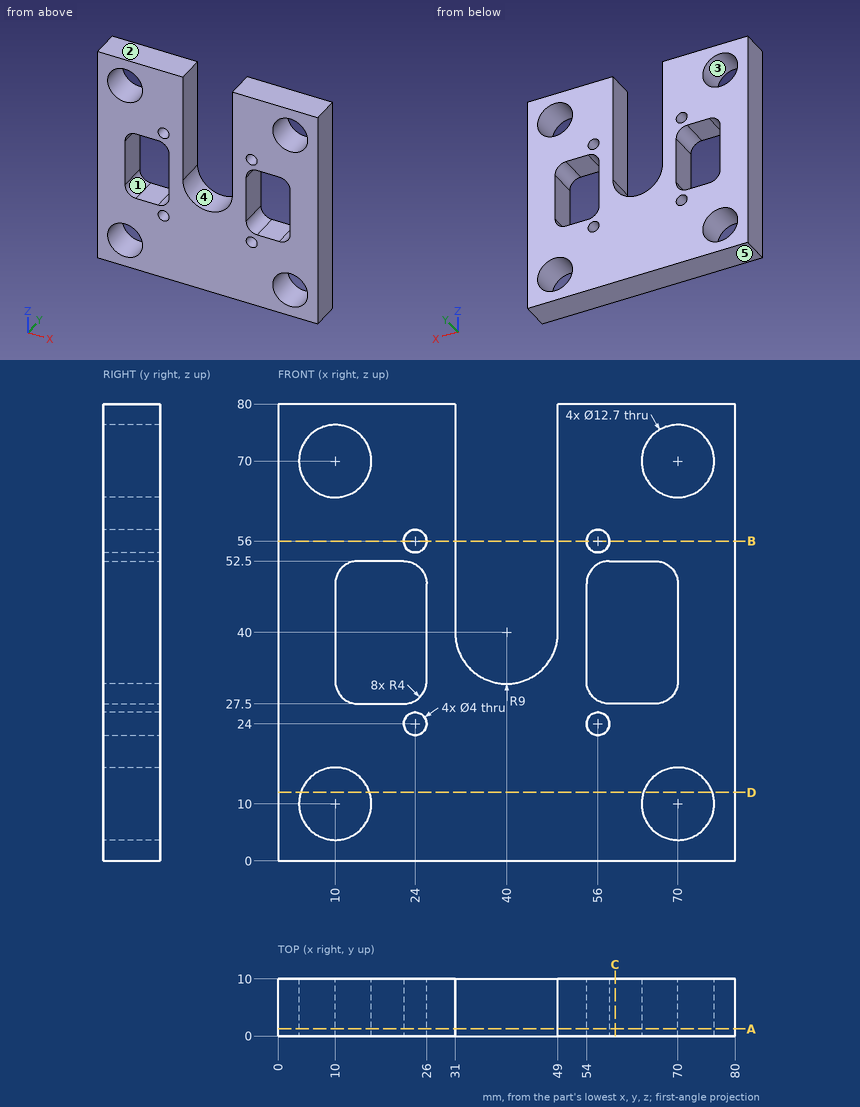
Design review of the part shown in the three views and the two pictorial views. Dimensions are in mm from the part's minimum x, y and z. A direction names the side the tool comes from. Round coordinates to 2 decimals unless told otherwise and drop trailing zeros. Write each loop counter-clockwise with the first axis right and the second up, starting at its lowest first coordinate (ties: lowest second). Pieces come first, ordered by that corner, then holes.
Item 1: The part is to be moulded in two halves that separate along Z. For the marked faces 3, 4 and 5, say which applies: +Z half, -Z half, draft (parallel to the pull), parting line (faces both ways), or undercut.
Item 2: We need section C-C on x = 59. Write out the cut boundary in (y, z), and give its area (3 significant figures).
Item 3: For probe 1 along X at (y, z) = (4, 24); probe 2 along X at (y, z) = (6.5, 56); probe 3 along X at (y, z) = (2.5, 63), list the stretches that pass through material, from the lowest coordinate up.
Item 4: We need section B-B on z = 56. Write out the cut boundary in (x, y).
Item 5: We need section A-A on y = 1.25. State how many separate pieces and enclosed holes the cut face has, and give its area (3 significant figures).
Item 6: We need section D-D on z = 12. Write out the cut boundary in (x, y).
Item 7: For the marked faces 1 and 2, list the 3-axis set-ups (+Z, -Z, +X, -X, +Y, -Y) from which the entire face can be reached by the end or side of a thin tool; tool diameter is ignored.
Item 8: Clearance check with a flat-ended pin moving along its axis: pin 1 Ø1 at (x, y) = (44, 9) entering from +Z. State where the tip first meets the part, or that it passes through.
Returned:
1. face 3: undercut
1. face 4: +Z half
1. face 5: -Z half
2. outline: (0, 0) - (10, 0) - (10, 27.5) - (0, 27.5) - close; (0, 52.5) - (10, 52.5) - (10, 80) - (0, 80) - close
2. area: 550 mm2
3. probe 1: x = 0 to 22, 26 to 54, 58 to 80
3. probe 2: x = 0 to 22, 26 to 31, 49 to 54, 58 to 80
3. probe 3: x = 0 to 31, 49 to 80
4. outline: (0, 0) - (22, 0) - (22, 10) - (0, 10) - close; (26, 0) - (31, 0) - (31, 10) - (26, 10) - close; (49, 0) - (54, 0) - (54, 10) - (49, 10) - close; (58, 0) - (80, 0) - (80, 10) - (58, 10) - close
5. separate pieces: 1
5. enclosed holes: 10
5. area: 4,220 mm2
6. outline: (0, 0) - (3.97, 0) - (3.97, 10) - (0, 10) - close; (16.03, 0) - (63.97, 0) - (63.97, 10) - (16.03, 10) - close; (76.03, 0) - (80, 0) - (80, 10) - (76.03, 10) - close
7. face 1: +Y, -Y
7. face 2: +Z, +X, -X, +Y, -Y
8. pin 1: stops at z = 32.21
